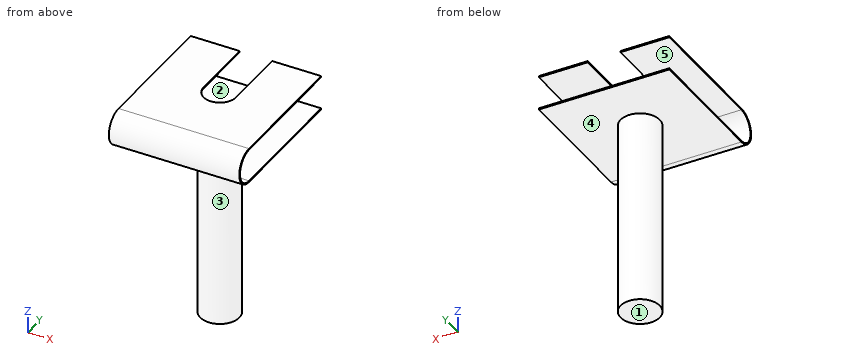
```python
from build123d import *

# Parameters (mm, degrees)
F1_DEPTH = 10
F3_DEPTH = 0.2
F4_R     = 3
F5_DEPTH = 30


with BuildPart() as f1:
    # F0 (on Right) → F1 (new body, symmetric)
    with BuildSketch(Plane.YZ):
        with BuildLine():
            Line((-10, 5), (10, 5))
            Line((10, 5), (10, 5.2))
            Line((10, 5.2), (-10, 5.2))
            ThreePointArc((-10, 5.2), (-12.7, 2.5), (-10, -0.2))
            Line((-10, -0.2), (10, -0.2))
            Line((10, -0.2), (10, 0))
            Line((10, 0), (-10, 0))
            ThreePointArc((-10, 0), (-12.5, 2.5), (-10, 5))
        make_face()
    extrude(amount=F1_DEPTH, both=True)

    # F2 (on face) → F3 (cut, through all)
    with BuildSketch(Plane.XY.offset(5.2)):
        with BuildLine():
            Line((-2.5, 10), (-2.5, 0))
            ThreePointArc((-2.5, 0), (0, -2.5), (2.5, 0))
            Line((2.5, 0), (2.5, 10))
            Line((2.5, 10), (-2.5, 10))
        make_face()
    extrude(amount=-F3_DEPTH, mode=Mode.SUBTRACT)

    # F4 (on face) → F5 (join)
    with BuildSketch(Plane(origin=(0, 0, -0.2), x_dir=(1, 0, 0), z_dir=(0, 0, -1))):
        Circle(F4_R)
    extrude(amount=F5_DEPTH)


solid = f1.part
```
The listing builds one solid part. Answer for the finished solid, in the listing's coordinates (mm). Face numbers are marked on the shaded views. A direction names the side the tool comes from. Give positions to 0.01 mm unless a question says otherwise; leave off trailing zeros. Order: outer loops, then holes, each group sorted by start corner. A loop starts at its lowest first (then second) coordinate and runs counter-clockwise, first axis right, second up. Notation, with made-up numbers: (71.5, -25) - (96.5, -25) arc R14 ccw to (96.5, -3) - close; hole circle Ø7 at (65, 76.25). An arc over 180 degrees is marked (long way). Answer in a Markdown table with one row per item. Add a question column.
Q1. The part is cut by section C-C (x = -4.5). Determine the outline of the cut face in (y, z), then the cut area to 3 significant figures.
Q2. The part is cut by section D-D (z = -9.5). Determine the outline of the cut face in (x, y).
Q3. The part is cut by section A-A (y = -3.5). Determine the outline of the cut face in (x, z).
Q4. For a pull along Z with two mould halves and no side action, classify the marked faces 3, 4 and 5 as released by +Z, released by -Z, zero draft, split by the parting line, or undercut.
Q5. Find the intervals of material crossed by line 1 along Z through (x, y) = (-3.5, 7.75); line 2 along Y through (x, z) = (-1, -19); line 3 along X through (y, z) = (-2, -26), in increasing order. Write a range as [from, to].
Q6. Which of the six approach directions +Z, -Z, +X, -X, +Y, -Y give full straight-line access (tool end or side, diameter ignored) to the marked faces 1 and 2?
Q7. The part is cut by section B-B (y = 6.25). Determine the outline of the cut face in (x, z).
Q8. Given P1, Ø4, axis at x = -3, y = -3, coming from the -Z side; P2, Ø10, axis at y = 7.5, z = -23.5, coming from the -X side; P3, Ø6, axis at x = 5.5, z = -9.5, coming from the +Y side; P4, Ø5, axis at y = 2, z = -3.5, coming from the -X side, each flat-ended and moving along its own axis, determine where each tip first touches the part or whether it passes through.
Determined:
| question | item | result |
|---|---|---|
| 1 | outline | (-10, -0.2) - (10, -0.2) - (10, 0) - (-10, 0) arc R2.5 cw to (-10, 5) - (10, 5) - (10, 5.2) - (-10, 5.2) arc R2.7 ccw to start |
| 1 | area | 9.63 mm² |
| 2 | outline | circle Ø6 at (0, 0) |
| 3 | outline | (-10, -0.2) - (10, -0.2) - (10, 0) - (-10, 0) - close; (-10, 5) - (10, 5) - (10, 5.2) - (-10, 5.2) - close |
| 4 | face 3 | zero draft |
| 4 | face 4 | released by -Z |
| 4 | face 5 | undercut |
| 5 | line 1 | z = [-0.2, 0], [5, 5.2] |
| 5 | line 2 | y = [-2.83, 2.83] |
| 5 | line 3 | x = [-2.24, 2.24] |
| 6 | face 1 | -Z, +X, -X, +Y, -Y |
| 6 | face 2 | +X, -X, +Y |
| 7 | outline | (-10, -0.2) - (10, -0.2) - (10, 0) - (-10, 0) - close; (-10, 5) - (-2.5, 5) - (-2.5, 5.2) - (-10, 5.2) - close; (2.5, 5) - (10, 5) - (10, 5.2) - (2.5, 5.2) - close |
| 8 | P1 | stops at z = -30.2 |
| 8 | P2 | stops at x = -1.66 |
| 8 | P3 | stops at y = 1.66 |
| 8 | P4 | stops at x = -3 |
